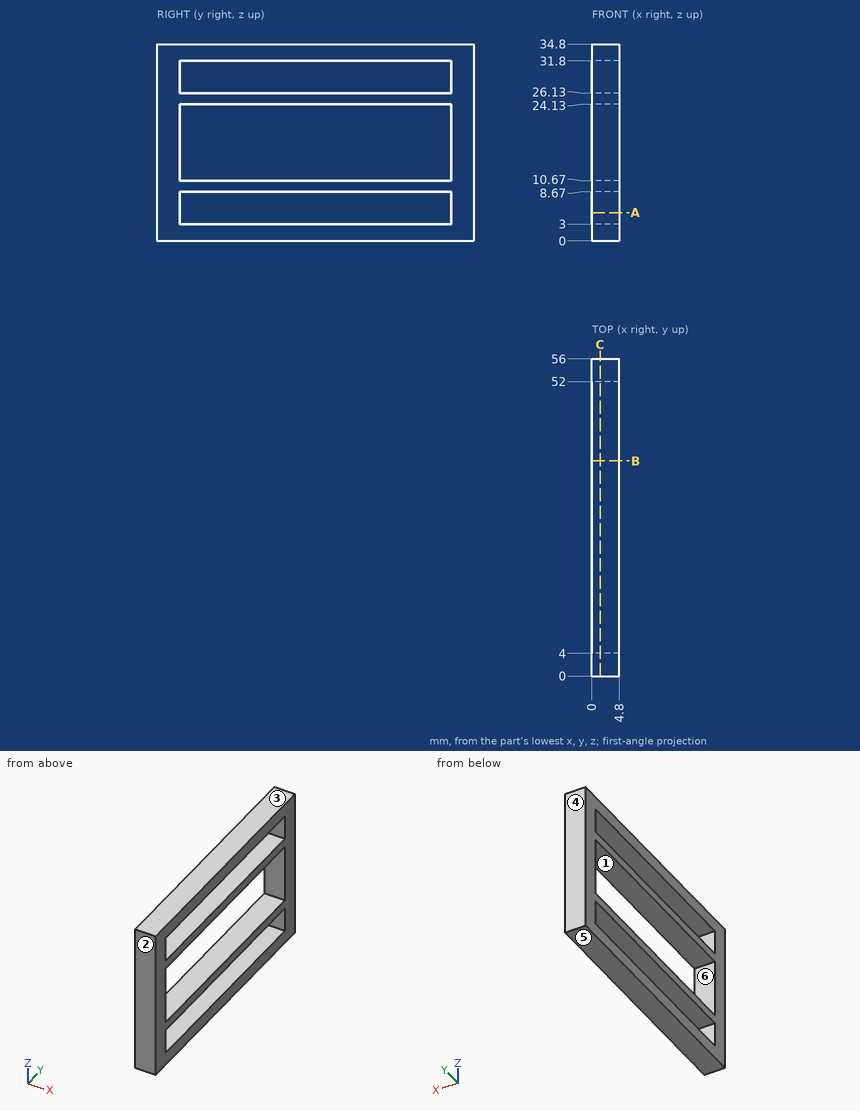
Design review of the part shown in the three views and the two pictorial views. Dimensions are in mm from the part's minimum x, y and z. A direction names the side the tool comes from. Coordinates: 2 decimals unless noted, no trailing zeros. Order: outer loops, then holes, each group sorted by start corner. A loop starts at its lowest first (then second) coordinate and runs counter-clockwise, first axis right, second up.
Item 1: For the marked faces 1 and 2, list the 3-axis set-ups (+Z, -Z, +X, -X, +Y, -Y) from which the entire face can be reached by the end or side of a thin tool; tool diameter is ignored.
Item 2: For line 1 (Z direction, x = 0.9, y = 25); line 2 (Y direction, x = 1.25, z = 15.5), list the stretches that pass through material, from the lowest coordinate up.
Item 3: Take a section at A-A, the plane z = 5. Write out the cut boundary in (x, y).
Item 4: Take a section at C-C, the plane x = 1.45. Write out the cut boundary in (y, z).
Item 5: Take a section at B-B, the plane y = 38. Write out the cut boundary in (x, z), then the cut area to 3 significant figures.
Item 6: The part is to be moulded in two halves that separate along Z. For the marked faces 3, 4, 5 and 6, say which applies: pulls with the +Z half, pulls with the -Z half, needs draft (parallel to the pull), parting line crosses it, or undercut.
The answers:
1. face 1: +X, -X
1. face 2: +Z, -Z, +X, -X, -Y
2. line 1: z = 0 to 3, 8.67 to 10.67, 24.13 to 26.13, 31.8 to 34.8
2. line 2: y = 0 to 4, 52 to 56
3. outline: (0, 0) - (4.8, 0) - (4.8, 4) - (0, 4) - close; (0, 52) - (4.8, 52) - (4.8, 56) - (0, 56) - close
4. outline: (0, 0) - (56, 0) - (56, 34.8) - (0, 34.8) - close; hole (4, 3) - (52, 3) - (52, 8.67) - (4, 8.67) - close; hole (4, 10.67) - (52, 10.67) - (52, 24.13) - (4, 24.13) - close; hole (4, 26.13) - (52, 26.13) - (52, 31.8) - (4, 31.8) - close
5. outline: (0, 0) - (4.8, 0) - (4.8, 3) - (0, 3) - close; (0, 8.67) - (4.8, 8.67) - (4.8, 10.67) - (0, 10.67) - close; (0, 24.13) - (4.8, 24.13) - (4.8, 26.13) - (0, 26.13) - close; (0, 31.8) - (4.8, 31.8) - (4.8, 34.8) - (0, 34.8) - close
5. area: 48.0 mm2
6. face 3: pulls with the +Z half
6. face 4: needs draft
6. face 5: pulls with the -Z half
6. face 6: undercut
